Could you check a few things on this model? Use its own coordinates, in mm. A direction names the side the tool comes from. Round coordinates to 2 decimals unless told otherwise and drop trailing zeros. Loops run counter-clockwise (first coordinate to the right, second up) from the corner with the lowest first, then second, coordinate; pieces in that order, holes last. Notation, with made-up numbers: (-17, 33.25) -> (32, 33.25) arc R30 cw to (32, 67.25) -> close; hole circle Ø2 at (-2, -3). An arc over 180 degrees is marked (long way). One line per item, written item: value.
from build123d import *

# Parameters (mm, degrees)
SKETCH_1_R          = 1.7
SKETCH_1_R_2        = 4
EXTRUDE_1_DEPTH     = 2
SKETCH_2_R          = 1.5
SKETCH_2_R_2        = 1.65
CUT_EXTRUDE_2_DEPTH = 86.626937008


with BuildPart() as part:
    # Эскиз1 → Бобышка-Вытянуть1 (new body)
    with BuildSketch(Plane(origin=(0, 0, 0), x_dir=(1, 0, 0), z_dir=(0, 1, 0))):
        with BuildLine():
            Line((-11.994516295, 0.362737998), (-27.997650279, 0.362737998))
            ThreePointArc((-27.997650279, 0.362737998), (-19.670324553, 19.926824433), (0, 28))
            ThreePointArc((0, 28), (10.111304648, 26.110563347), (18.857990039, 20.697251308))
            Line((18.857990039, 20.697251308), (47.343097909, -5.256527408))
            add(Edge.make_bspline(
                [(63.764396425, -54.631632015), (73.929390971, -32.189504173), (47.343097909, -5.256527408)],
                knots=[3.37709689, 3.37709689, 3.37709689, 4.71238898, 4.71238898, 4.71238898], degree=2, weights=[1, 0.785281266, 1]))
            Line((63.764396425, -54.631632015), (58.046409316, -48.83908269))
            add(Edge.make_bspline(
                [(58.046409316, -48.83908269), (65.599461261, -3.0612118), (10.459692489, 5.881737247)],
                knots=[0.348473456, 0.348473456, 0.348473456, 2.541551794, 2.541551794, 2.541551794], degree=2, weights=[1, 0.456677717, 1]))
            ThreePointArc((10.459692489, 5.881737247), (2.864220523, -11.653164411), (-11.994516295, 0.362737998))
        make_face()
        with Locations(Location((-6.322604321, 6.40505071, 0), (0, 0, 270))):
            Circle(SKETCH_1_R, mode=Mode.SUBTRACT)
        with Locations(Location((0, 0, 0), (0, 0, 270))):
            Circle(SKETCH_1_R_2, mode=Mode.SUBTRACT)
        with Locations(Location((8.708238788, 2.273010605, 0), (0, 0, 270))):
            Circle(SKETCH_1_R, mode=Mode.SUBTRACT)
        with Locations(Location((-2.385634467, -8.678061315, 0), (0, 0, 270))):
            Circle(SKETCH_1_R, mode=Mode.SUBTRACT)
    extrude(amount=EXTRUDE_1_DEPTH)

    # Эскиз2 → Вырез-Вытянуть2 (cut, through all)
    with BuildSketch(Plane(origin=(0, 2, 0), x_dir=(1, 0, 0), z_dir=(0, 1, 0))):
        with Locations(Location((-4.341204442, 24.620193825, 0), (0, 0, 270))):
            Circle(SKETCH_2_R)
        with Locations(Location((-14.339410909, 20.478801107, 0), (0, 0, 90))):
            Circle(SKETCH_2_R)
        with Locations(Location((51.61994824, -19.642751406, 0), (0, 0, 270))):
            Circle(SKETCH_2_R_2)
        with Locations(Location((61.034534355, -39.343644659, 0), (0, 0, 270))):
            Circle(SKETCH_2_R_2)
        with Locations(Location((33.013487472, -0.79366348, 0), (0, 0, 270))):
            Circle(SKETCH_2_R_2)
    extrude(amount=-CUT_EXTRUDE_2_DEPTH, mode=Mode.SUBTRACT)


solid = part.part
(1) Thinking about a two-plate mould opening in X: for faces 3 (the face through (32.901, 0.986, -7.902)), 4 (the face through (50.988, 1.014, 21.167)), 5 (the face through (16, 2, -5)), which applies, released by +X, released by -X, zero draft, split by the parting line, or undercut?
Recorded:
face 3: released by +X
face 4: undercut
face 5: zero draft
(2) I'm going to push flat-ended pins straight in: pin 1 Ø5 at (x, z) = (-4.34, -24.62) entering from -Y; pin 2 Ø1 at (x, y) = (-17, 1) entering from +Z; pin 3 Ø1 at (y, z) = (1.5, 2) entering from -X. Where does each tip first touch, or does it pass through?
Recorded:
pin 1: y = 0
pin 2: z = -0.36
pin 3: x = -11.91
(3) If I drill on L1, parallel to Z at x = 32, y = 0.65; L2, parallel to X at y = 1.4, z = -3; L3, parallel to Z at x = 10, y = 1.85, over which ranges is the centre line in solid material (lowest first)?
Recorded:
L1: -8.72 to -0.51, 2.1 to 4.39
L2: -27.84 to -2.65, 2.65 to 7.17, 10.24 to 11.62, 19.71 to 38.28
L3: -26.15 to -3.38, -1.17 to 6.63
(4) For faces 1 (the face through (61.107, 1.014, 37.695)), 2 (the face through (-20, 1, -0.363)), which set-ups out of +Z, -Z, +X, -X, +Y, -Y let a thin tool reach every point of the face, with its end or its side?
Recorded:
face 1: +Y, -Y
face 2: +Z, -X, +Y, -Y
(5) If we section it at B-B, the plane x = -9.5: Please give me the cut outline in (y, z), then the cut area to 3 significant figures.
Recorded:
outline: (0, -26.34) -> (2, -26.34) -> (2, 7.33) -> (0, 7.33) -> close
area: 67.3 mm²
(6) If we section it at A-A, the plane x = 1.5: Please give me the cut outline in (y, z), then the cut area to 3 significant figures.
Recorded:
outline: (0, -27.96) -> (2, -27.96) -> (2, -3.71) -> (0, -3.71) -> close; (0, 3.71) -> (2, 3.71) -> (2, 11.91) -> (0, 11.91) -> close
area: 64.9 mm²
